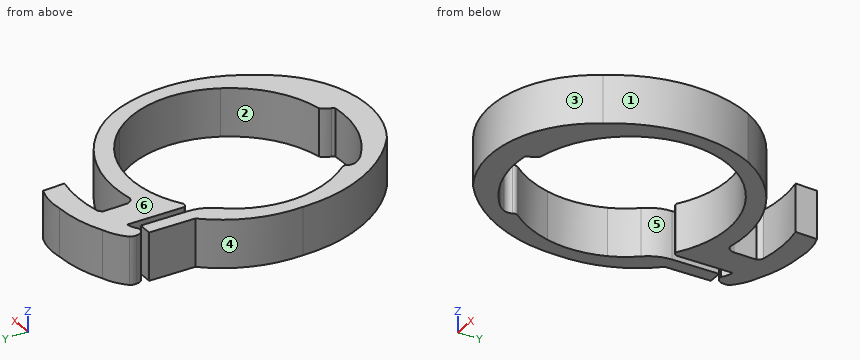
```python
from build123d import *

# Parameters (mm, degrees)
BOSS_EXTRUDE1_DEPTH = 11


with BuildPart() as part:
    # Sketch1 → Boss-Extrude1 (new body)
    with BuildSketch(Plane.XY):
        with BuildLine():
            Line((-18.853830773, 25.160435071), (-16.119000888, 25.233110696))
            Line((-16.119000888, 25.233110696), (-16.119000888, 14.613334924))
            ThreePointArc((-16.119000888, 14.613334924), (-16.64958264, 11.530072447), (-18.180286861, 8.801525384))
            ThreePointArc((-18.180286861, 8.801525384), (-20.022572688, 6.105775505), (-21.399060798, 3.144970722))
            ThreePointArc((-21.399060798, 3.144970722), (-22.726569744, -3.354769567), (-22.053552104, -9.954462823))
            ThreePointArc((-22.053552104, -9.954462823), (-20.106400366, -15.071180428), (-17.085436321, -19.636919707))
            ThreePointArc((-17.085436321, -19.636919707), (-16.826323912, -20.249507523), (-16.951603049, -20.902736587))
            ThreePointArc((-16.951603049, -20.902736587), (-17.18386468, -21.838882371), (-16.955503917, -22.775987357))
            ThreePointArc((-16.955503917, -22.775987357), (-16.236029845, -23.865360174), (-15.307939029, -24.783523292))
            ThreePointArc((-15.307939029, -24.783523292), (-6.902922169, -29.070783982), (2.514195466, -29.656282157))
            ThreePointArc((2.514195466, -29.656282157), (2.798104907, -29.369092957), (2.954895281, -28.996938438))
            ThreePointArc((2.954895281, -28.996938438), (3.387996909, -27.87172525), (4.151482129, -26.938573569))
            ThreePointArc((4.151482129, -26.938573569), (13.70577614, -22.445002036), (20.325671696, -14.219814986))
            ThreePointArc((20.325671696, -14.219814986), (22.482847249, -1.351664436), (17.013236546, 10.494265824))
            ThreePointArc((17.013236546, 10.494265824), (2.522103549, 17.974028049), (-13.285319782, 13.96589306))
            ThreePointArc((-13.285319782, 13.96589306), (-14.010252719, 14.025446056), (-14.438576198, 14.613334924))
            Line((-14.438576198, 14.613334924), (-14.463639713, 27.310804635))
            ThreePointArc((-14.463639713, 27.310804635), (-15.772674476, 26.882496645), (-16.921609527, 26.122912554))
            ThreePointArc((-16.921609527, 26.122912554), (-18.247717994, 26.438122976), (-18.831203914, 27.669977456))
            ThreePointArc((-18.831203914, 27.669977456), (-18.868217492, 28.483440244), (-18.573500133, 29.242540627))
            ThreePointArc((-18.573500133, 29.242540627), (-16.413121418, 31.153842986), (-13.848257568, 32.473610515))
            ThreePointArc((-13.848257568, 32.473610515), (-8.344696861, 34.627822793), (-2.50820992, 35.558000832))
            ThreePointArc((-2.50820992, 35.558000832), (1.150912858, 35.75032292), (4.737729096, 35.001379281))
            Line((4.737729096, 35.001379281), (4.992549443, 30.035082131))
            ThreePointArc((4.992549443, 30.035082131), (-0.915054965, 30.467339098), (-6.792394138, 29.7301009))
            ThreePointArc((-6.792394138, 29.7301009), (-7.409462923, 29.370020494), (-7.826896167, 28.790209084))
            Line((-7.826896167, 28.790209084), (-7.712079502, 23.601110726))
            ThreePointArc((-7.712079502, 23.601110726), (-7.280949637, 22.466131343), (-6.230949855, 21.856581002))
            ThreePointArc((-6.230949855, 21.856581002), (10.429887602, 20.043351617), (22.848599934, 8.789601594))
            ThreePointArc((22.848599934, 8.789601594), (26.218834648, -7.288142965), (20.968539738, -22.853706092))
            ThreePointArc((20.968539738, -22.853706092), (6.607574044, -34.777230529), (-11.948618389, -32.758445472))
            ThreePointArc((-11.948618389, -32.758445472), (-22.400695848, -20.847022299), (-26.08676765, -5.434663624))
            ThreePointArc((-26.08676765, -5.434663624), (-24.658208176, 5.345172428), (-19.217331386, 14.760187417))
            Line((-19.217331386, 14.760187417), (-19.177343822, 25.15499714))
            Line((-19.177343822, 25.15499714), (-18.853830773, 25.160435071))
        make_face()
    extrude(amount=BOSS_EXTRUDE1_DEPTH)


solid = part.part
```
Check sheet for the modelled part. Datum: model origin and axes. Units: mm. Face numbers are marked on the shaded views. A direction names the side the tool comes from. Round coordinates to 2 decimals unless told otherwise and drop trailing zeros. Order: outer loops, then holes, each group sorted by start corner. A loop starts at its lowest first (then second) coordinate and runs counter-clockwise, first axis right, second up.
1) Tool access check on the marked faces 1 and 2. Record the directions out of +Z, -Z, +X, -X, +Y, -Y that give a thin tool (end or side, any length) a straight path to the whole face; none if there is none.
2) Scan lines: line 1 (Y direction, x = -3, z = 9.5); line 2 (Y direction, x = 4, z = 2.25); line 3 (X direction, y = 10, z = 8). Record each from-to range of solid material in increasing order.
3) Section check B-B (y = 19). Record the boundary of the cut face in (x, z), and give its area (3 significant figures).
4) Section check A-A (x = 10.5). Record the boundary of the cut face in (y, z), and give its area (3 significant figures).
5) Mould release check, pull along X, two halves, no side actions. Record for the marked faces 3, 4, 5 and 6: +X half, -X half, draft (parallel to the pull), parting line (faces both ways), or undercut.
6) Go/stop test with flat-tipped pins: pin 1 Ø4 at (y, z) = (4.5, 9) entering from -X; pin 2 Ø5 at (y, z) = (14, 2.5) entering from -X; pin 3 Ø1 at (x, z) = (13.5, 6) entering from +Y. Record where each tip stops, or that it passes through.
Result:
1. face 1: +Z, -Z, +X
1. face 2: +Z, -Z
2. line 1: y = -35.64 to -29.79, 17.94 to 22.33, 30.34 to 35.53
2. line 2: y = -35.4 to -27.08, 17.76 to 22.02, 30.19 to 35.24
2. line 3: x = -22.58 to -17.36, 17.44 to 22.11
3. outline: (-19.2, 0) - (-16.12, 0) - (-16.12, 11) - (-19.2, 11) - close; (-14.45, 0) - (12.51, 0) - (12.51, 11) - (-14.45, 11) - close
3. area: 330 mm2
4. outline: (-33.22, 0) - (-24.57, 0) - (-24.57, 11) - (-33.22, 11) - close; (15.54, 0) - (20.01, 0) - (20.01, 11) - (15.54, 11) - close
4. area: 144 mm2
5. face 3: parting line
5. face 4: -X half
5. face 5: undercut
5. face 6: draft
6. pin 1: stops at x = -25.46
6. pin 2: stops at x = -21.68
6. pin 3: stops at y = 18.72
